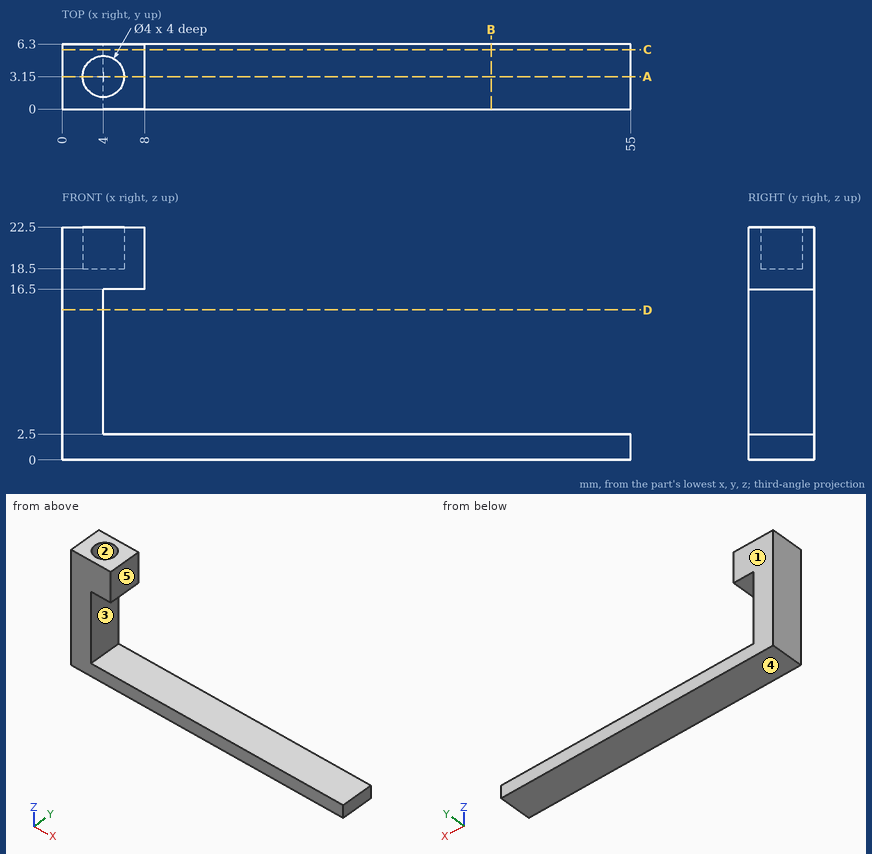
Geometry check sheet. Reference: drawing and pictorial views, mm from the part's lowest x, y, z. A direction names the side the tool comes from. Round coordinates to 2 decimals unless told otherwise and drop trailing zeros. Order: outer loops, then holes, each group sorted by start corner. A loop starts at its lowest first (then second) coordinate and runs counter-clockwise, first axis right, second up. Notation, with made-up numbers: M 1.25,53 L 23.25,53 A12 cw 23.25,60 Z; hole C -20,-23.75 d2. An arc over 180 degrees is marked long. Write item = value, one per line.
Q1. Section check D-D (z = 14.5). Enter the section's corners in (x, y).
Answer block:
outline = M 0,0 L 4,0 L 4,6.3 L 0,6.3 Z
Q2. Depth check by flat-ended pin: pin 1 Ø1.2 at (x, y) = (3, 4) entering from +Z; pin 2 Ø3 at (x, y) = (31.5, 2.5) entering from +Z; pin 3 Ø3 at (y, z) = (2.5, 12.5) entering from +X; pin 4 Ø10 at (x, z) = (15.5, 19) entering from +Y. Enter the tip coordinate at first touch or a pass-through.
Answer block:
pin_1 = 18.5
pin_2 = 2.5
pin_3 = 4
pin_4 = through
Q3. Scan lines: line 1 (X direction, y = 3.15, z = 21.4); line 2 (Y direction, x = 4, z = 19.45); line 3 (X direction, y = 4, z = 9.75). Record each from-to range of solid material in increasing order.
Answer block:
line_1 = 0 to 2, 6 to 8
line_2 = 0 to 1.15, 5.15 to 6.3
line_3 = 0 to 4
Q4. Release check for a two-part mould opening along Z. For the marked faces 3, 4 and 5 record: released by +Z, released by -Z, zero draft, split by the parting line, or undercut.
Answer block:
face_3 = undercut
face_4 = released by -Z
face_5 = zero draft
Q5. Section check C-C (y = 5.75). Enter the section's corners in (x, z), plus the area to 4 significant figures.
Answer block:
outline = M 0,0 L 55,0 L 55,2.5 L 4,2.5 L 4,16.5 L 8,16.5 L 8,22.5 L 0,22.5 Z
area = 241.5 mm^2
Q6. Set-up check for the marked faces 1 and 2: record each of +Z, -Z, +X, -X, +Y, -Y from which the full face is reachable in a straight line by a thin tool's end or side.
Answer block:
face_1 = +Z, -Z, +X, -X, +Y
face_2 = +Z
Q7. Section check B-B (x = 41.5). Enter the section's corners in (y, z).
Answer block:
outline = M 0,0 L 6.3,0 L 6.3,2.5 L 0,2.5 Z
Q8. Section check A-A (y = 3.15). Enter the section's corners in (x, z), plus the area to 4 significant figures.
Answer block:
outline = M 0,0 L 55,0 L 55,2.5 L 4,2.5 L 4,16.5 L 8,16.5 L 8,22.5 L 6,22.5 L 6,18.5 L 2,18.5 L 2,22.5 L 0,22.5 Z
area = 225.5 mm^2
